```python
from build123d import *

# Parameters (mm, degrees)
SKETCH1_R           = 1.5
BOSS_EXTRUDE1_DEPTH = 22.5
CUT_EXTRUDE1_DEPTH  = 10
CUT_EXTRUDE2_DEPTH  = 10


with BuildPart() as part:
    # Sketch1 → Boss-Extrude1 (new body, symmetric)
    with BuildSketch(Plane(origin=(0, 0, 0), x_dir=(0, 0, -1), z_dir=(1, 0, 0))):
        Circle(SKETCH1_R)
    extrude(amount=BOSS_EXTRUDE1_DEPTH, both=True)

    # Sketch2 → Cut-Extrude1 (cut)
    with BuildSketch(Plane(origin=(22.5, 0, 0), x_dir=(0, 0, -1), z_dir=(1, 0, 0))):
        with BuildLine():
            Line((1.118033989, 1), (-1.118033989, 1))
            ThreePointArc((-1.118033989, 1), (0, 1.5), (1.118033989, 1))
        make_face()
    extrude(amount=-CUT_EXTRUDE1_DEPTH, mode=Mode.SUBTRACT)

    # Sketch3 → Cut-Extrude2 (cut)
    with BuildSketch(Plane(origin=(22.5, 0, 0), x_dir=(0, 0, -1), z_dir=(1, 0, 0))):
        with BuildLine():
            Line((1.118033989, 1), (1.118033989, -1))
            ThreePointArc((1.118033989, -1), (1.5, 0), (1.118033989, 1))
        make_face()
    extrude(amount=-CUT_EXTRUDE2_DEPTH, mode=Mode.SUBTRACT)


solid = part.part
```
Check sheet for the modelled part. Datum: model origin and axes. Units: mm. A direction names the side the tool comes from. Give positions to 0.01 mm unless a question says otherwise; leave off trailing zeros. Write each loop counter-clockwise with the first axis right and the second up, starting at its lowest first coordinate (ties: lowest second). Pieces come first, ordered by that corner, then holes. Notation, with made-up numbers: (58, -19.5) - (110, -19.5) arc R28 ccw to (110, -1.5) - close; hole circle Ø9 at (28.25, 7). An arc over 180 degrees is marked (long way). Answer as a JSON object with one key per item and string values. Group by question number.
1) Sectioned sample at A-A (z = 0). Record the cut outline in (x, y).
2) Access from +Z, -Z, +X, -X, +Y, -Y to the whole of each face (thin tool, end or side, straight path). Record for faces 1 (the face through (18, 1, 0)), 2 (the face through (18, 0, -1.118)), 3 (the face through (0.315, -1.464, 0.325)).
3) Thickness scan on probe 1 along Z at (x, y) = (-15, -1.25); probe 2 along Z at (x, y) = (1, -1); probe 3 along Y at (x, z) = (7.5, 1.35). Record the ranges inside material, lowest first. Write a range as from..to.
4) Sectioned sample at B-B (y = 0). Record the cut outline in (x, z), then the cut area to 3 significant figures.
5) Depth check by flat-ended pin: P1, Ø1.5, axis at x = 11.5, z = -1, coming from the +Y side. Enter the tip coordinate at first touch or a pass-through.
6) Sectioned sample at C-C (x = -1.5). Record the cut outline in (y, z), then the cut area to 3 significant figures.
Geometry results:
{
 "1": {"outline": "(-22.5, -1.5) - (22.5, -1.5) - (22.5, 1) - (12.5, 1) - (12.5, 1.5) - (-22.5, 1.5) - close"},
 "2": {"face 1": "+Z, -Z, +X, +Y", "face 2": "-Z, +X, +Y, -Y", "face 3": "+X, -X"},
 "3": {"probe 1": "z = -0.83..0.83", "probe 2": "z = -1.12..1.12", "probe 3": "y = -0.65..0.65"},
 "4": {"outline": "(-22.5, -1.5) - (12.5, -1.5) - (12.5, -1.12) - (22.5, -1.12) - (22.5, 1.5) - (-22.5, 1.5) - close", "area": "131 mm^2"},
 "5": {"P1": "stops at y = 1.48"},
 "6": {"outline": "circle Ø3 at (0, 0)", "area": "7.07 mm^2"}
}
